from build123d import *

# Parameters (mm, degrees)
SKETCH1_R           = 48
SKETCH1_R_2         = 23.5
SKETCH1_R_3         = 4
BOSS_EXTRUDE1_DEPTH = 10
CUT_EXTRUDE3_START  = -2
SKETCH2_R           = 25
SKETCH2_R_2         = 23.5
CUT_EXTRUDE3_DEPTH  = 2
CUT_EXTRUDE4_DEPTH  = 11
CIRPATTERN4_COUNT   = 4
SKETCH4_R           = 25.5
SKETCH4_R_2         = 21.5
BOSS_EXTRUDE2_DEPTH = 5
FILLET1_R           = 2
FILLET2_R           = 1


with BuildPart() as part:
    # Sketch1 → Boss-Extrude1 (new body)
    with BuildSketch(Plane.XY):
        Circle(SKETCH1_R)
        Circle(SKETCH1_R_2, mode=Mode.SUBTRACT)
        with Locations((37.5, 0)):
            Circle(SKETCH1_R_3, mode=Mode.SUBTRACT)
        with Locations((0, 37.5)):
            Circle(SKETCH1_R_3, mode=Mode.SUBTRACT)
        with Locations((-37.5, 0)):
            Circle(SKETCH1_R_3, mode=Mode.SUBTRACT)
        with Locations((0, -37.5)):
            Circle(SKETCH1_R_3, mode=Mode.SUBTRACT)
    extrude(amount=BOSS_EXTRUDE1_DEPTH)

    # Sketch2 → Cut-Extrude3 (cut)
    with BuildSketch(Plane.XY.offset(10).offset(CUT_EXTRUDE3_START)):
        Circle(SKETCH2_R)
        Circle(SKETCH2_R_2, mode=Mode.SUBTRACT)
    extrude(amount=-CUT_EXTRUDE3_DEPTH, mode=Mode.SUBTRACT)

    # Sketch3 → Cut-Extrude4 (cut, through all)
    with BuildSketch(Plane(origin=(0, 0, 0), x_dir=(-1, 0, 0), z_dir=(0, 0, -1))):
        with BuildLine():
            Line((-9.741058681, 41.419410131), (-17.239305551, 22.783732741))
            ThreePointArc((-17.239305551, 22.783732741), (-19.445436483, 19.445436483), (-22.783732741, 17.239305551))
            Line((-22.783732741, 17.239305551), (-41.419410131, 9.741058681))
            ThreePointArc((-41.419410131, 9.741058681), (-46.200684064, 5.877762909), (-48, 0))
            ThreePointArc((-48, 0), (-33.941125497, 33.941125497), (0, 48))
            ThreePointArc((0, 48), (-5.877762909, 46.200684064), (-9.741058681, 41.419410131))
        make_face()
    cut_extrude4 = extrude(amount=-CUT_EXTRUDE4_DEPTH, mode=Mode.SUBTRACT)

    # CirPattern4: Cut-Extrude4 ×4 about axis
    cirpattern4_axis = Axis((0, 0, 0), (0, 0, 1))
    for i in range(1, CIRPATTERN4_COUNT):
        add(cut_extrude4.rotate(cirpattern4_axis, i * 360 / CIRPATTERN4_COUNT), mode=Mode.SUBTRACT)

    # Sketch4 → Boss-Extrude2 (add)
    with BuildSketch(Plane(origin=(0, 0, 0), x_dir=(-1, 0, 0), z_dir=(0, 0, -1))):
        Circle(SKETCH4_R)
        Circle(SKETCH4_R_2, mode=Mode.SUBTRACT)
    extrude(amount=BOSS_EXTRUDE2_DEPTH)

    # Fillet1
    fillet1_edges = [part.edges().sort_by_distance(p)[0] for p in [
        (25.5, 0, -5),
    ]]
    fillet(fillet1_edges, radius=FILLET1_R)

    # Fillet2
    fillet2_edges = [part.edges().sort_by_distance(p)[0] for p in [
        (25.5, 0, 0),
    ]]
    fillet(fillet2_edges, radius=FILLET2_R)


solid = part.part
Design review of the part built by this model. Coordinates are the model's own, in mm. A direction names the side the tool comes from. Coordinates: 2 decimals unless noted, no trailing zeros. Loops run counter-clockwise (first coordinate to the right, second up) from the corner with the lowest first, then second, coordinate; pieces in that order, holes last. Notation, with made-up numbers: M 28.25,-29 L 58.25,-29 A35 cw 58.25,8 Z; hole C 41,25 d5. An arc over 180 degrees is marked long. Answer as CSV lines item,"result".
Item 1: For P1, Ø1, axis at y = 30, z = 4.5, coming from the +X side; P2, Ø15, axis at x = 8.5, y = 4, coming from the -Z side; P3, Ø13, axis at x = 0, y = 37.5, coming from the -Z side; P4, Ø4, axis at y = -27.5, z = 0.5, coming from the +X side, all flat-tipped, find the tip position at first contact; note any pin that passes through.
Answer list:
P1,"x = 14.54"
P2,"through"
P3,"z = 0"
P4,"x = 16.15"
Item 2: Machinability: for faces 1 (the face through (-17, -17, 6)), 2 (the face through (25, -10, 0)), 3 (the face through (22.4, 7.1, 3)), which of the approach directions +Z, -Z, +X, -X, +Y, -Y give a long, thin tool a straight path to every point of the face, cutting with its end or side? Answer none if there is none.
Answer list:
face 1,"none"
face 2,"-Z"
face 3,"+Z"
Item 3: Add section C-C on x = 37.5. State the section outline as (y, z) points, plus the area to 3 significant figures.
Answer list:
outline,"M -11.32,0 L -4,0 L -4,10 L -11.32,10 Z; M 4,0 L 11.32,0 L 11.32,10 L 4,10 Z"
area,"146 mm²"
Item 4: The part is to be moulded in two halves that separate along X. For faces 4 (the face through (-0.521, 41.466, 4.93)), 5 (the face through (19.406, 19.485, 4.93)), 6 (the face through (-11, -21, 10)), 7 (the face through (23.846, 7.509, 7.014)), say which applies: pulls with the +X half, pulls with the -X half, needs draft (parallel to the pull), parting line crosses it, or undercut.
Answer list:
face 4,"undercut"
face 5,"pulls with the +X half"
face 6,"needs draft"
face 7,"undercut"
Item 5: For probe 1 along Y at (x, z) = (-39.5, 8.5); probe 2 along Y at (x, z) = (-14, 1.5); probe 3 along Z at (x, y) = (30, 10), list the stretches that pass through material, from the lowest coordinate up.
Answer list:
probe 1,"-10.51 to -3.46, 3.46 to 10.51"
probe 2,"-30.83 to -18.87, 18.87 to 30.83"
probe 3,"0 to 10"
Item 6: Add section A-A on z = 1.75. State the section outline as (x, y) points, plus the area to 3 significant figures.
Answer list:
outline,"M -41.42,-9.74 L -22.78,-17.24 A10 cw -17.24,-22.78 L -9.74,-41.42 A10.5 ccw 9.74,-41.42 L 17.24,-22.78 A10 cw 22.78,-17.24 L 41.42,-9.74 A10.5 ccw 41.42,9.74 L 22.78,17.24 A10 cw 17.24,22.78 L 9.74,41.42 A10.5 ccw -9.74,41.42 L -17.24,22.78 A10 cw -22.78,17.24 L -41.42,9.74 A10.5 ccw Z; hole C -37.5,0 d8; hole C 0,0 d47; hole C 0,-37.5 d8; hole C 0,37.5 d8; hole C 37.5,0 d8"
area,"2,440 mm²"
Item 7: Add section B-B on y = 36. State the section outline as (x, z) points, plus the area to 3 significant figures.
Answer list:
outline,"M -11.92,0 L -3.71,0 L -3.71,10 L -11.92,10 Z; M 3.71,0 L 11.92,0 L 11.92,10 L 3.71,10 Z"
area,"164 mm²"
